Geometry check sheet. Reference: the model listing, model coordinates, mm. A direction names the side the tool comes from. Give positions to 0.01 mm unless a question says otherwise; leave off trailing zeros. Loops run counter-clockwise (first coordinate to the right, second up) from the corner with the lowest first, then second, coordinate; pieces in that order, holes last. Notation, with made-up numbers: (30, -0.5) -> (47, -0.5) arc R11 ccw to (47, 8.5) -> close; hole circle Ø9 at (53, 74.5). An arc over 180 degrees is marked (long way). One line per item, written item: value. Start each with the question number.
(1) Sectioned sample at B-B, the plane y = 25. Record the cut outline in (x, z).
(2) Sectioned sample at C-C, the plane z = 0. Record the cut outline in (x, y), then the cut area to 3 significant figures.
(3) Tool access check on faces 1 (the face through (0, 29, -16)), 2 (the face through (-22.7, 29.7, -10)), 3 (the face through (36, 8, 7.276)). Record the directions out of +Z, -Z, +X, -X, +Y, -Y that give a thin tool (end or side, any length) a straight path to the whole face; none if there is none.
(4) Scan lines: line 1 along Z through (x, y) = (-13, 40); line 2 along X through (y, z) = (40, -16.5); line 3 along Y through (x, z) = (-24, 14.5). Record each from-to range of solid material in increasing order. Write a range as from..to.
(5) Sectioned sample at A-A, the plane x = -24. Record the cut outline in (y, z).
(6) Gauge pin test, flat ends, axial feed: pin 1 Ø9.5 at (y, z) = (32.5, -14.5) entering from +X; pin 2 Ø2 at (x, z) = (-1, -11) entering from +Y; pin 3 Ø2 at (x, z) = (29.5, 10) entering from +Y; pin 4 Ø8 at (y, z) = (27, -3.5) entering from +X. Record the tip position at first contact, or that the pin passes through.
(7) Sectioned sample at D-D, the plane z = -19. Record the cut outline in (x, y).
(8) Draft check along X on faces 4 (the face through (-48, 15, 0)), 5 (the face through (12, 16, 0)), 6 (the face through (16.725, 7.888, 0.16)). Enter one of: pulls with the +X half, pulls with the -X half, needs draft (parallel to the pull), parting line crosses it, or undercut.
from build123d import *

# Parameters (mm, degrees)
BOSS_EXTRUDE1_DEPTH = 16
CUT_EXTRUDE2_DEPTH  = 16
SKETCH3_R           = 10
BOSS_EXTRUDE2_DEPTH = 12
BOSS_EXTRUDE3_START = -12
SKETCH11_R          = 10
BOSS_EXTRUDE3_DEPTH = 12
FILLET1_R           = 2
FILLET2_R           = 2


with BuildPart() as part:
    # Sketch1 → Boss-Extrude1 (new body)
    with BuildSketch(Plane(origin=(0, 0, 0), x_dir=(1, 0, 0), z_dir=(0, 1, 0))):
        with BuildLine():
            Line((-48, 22), (48, 22))
            ThreePointArc((48, 22), (70, 0), (48, -22))
            Line((48, -22), (-48, -22))
            Line((-48, -22), (-48, 22))
        make_face()
    extrude(amount=BOSS_EXTRUDE1_DEPTH)

    # Sketch2 → Cut-Extrude2 (cut)
    with BuildSketch(Plane(origin=(0, 0, 0), x_dir=(1, 0, 0), z_dir=(0, 1, 0))):
        with BuildLine():
            Line((48, -7.276334806), (24, -7.276334806))
            ThreePointArc((24, -7.276334806), (16.723665194, 0), (24, 7.276334806))
            Line((24, 7.276334806), (48, 7.276334806))
            ThreePointArc((48, 7.276334806), (55.276334806, 0), (48, -7.276334806))
        make_face()
    extrude(amount=CUT_EXTRUDE2_DEPTH, mode=Mode.SUBTRACT)

    # Sketch3 → Boss-Extrude2 (add)
    with BuildSketch(Plane.XY.offset(22)):
        with BuildLine():
            Line((-48, 40), (-48, 16))
            Line((-48, 16), (0, 16))
            Line((0, 16), (0, 40))
            ThreePointArc((0, 40), (-24, 64), (-48, 40))
        make_face()
        with Locations((-24, 40)):
            Circle(SKETCH3_R, mode=Mode.SUBTRACT)
    extrude(amount=-BOSS_EXTRUDE2_DEPTH)

    # Sketch11 → Boss-Extrude3 (add)
    with BuildSketch(Plane(origin=(0, 0, -22), x_dir=(-1, 0, 0), z_dir=(0, 0, -1)).offset(BOSS_EXTRUDE3_START)):
        with BuildLine():
            Line((0, 16), (48, 16))
            Line((48, 16), (48, 40))
            ThreePointArc((48, 40), (24, 64), (0, 40))
            Line((0, 40), (0, 16))
        make_face()
        with Locations(Location((24, 40, 0), (0, 0, 180))):
            Circle(SKETCH11_R, mode=Mode.SUBTRACT)
    extrude(amount=BOSS_EXTRUDE3_DEPTH)

    # Fillet1
    fillet1_edges = [part.edges().sort_by_distance(p)[0] for p in [
        (0, 16, 16),
    ]]
    fillet(fillet1_edges, radius=FILLET1_R)

    # Fillet2
    fillet2_edges = [part.edges().sort_by_distance(p)[0] for p in [
        (0, 16, -16),
    ]]
    fillet(fillet2_edges, radius=FILLET2_R)


solid = part.part
Calculated:
1. outline: (-48, -22) -> (0, -22) -> (0, -10) -> (-48, -10) -> close; (-48, 10) -> (0, 10) -> (0, 22) -> (-48, 22) -> close
2. outline: (-48, 0) -> (16.72, 0) -> (16.72, 16) -> (-48, 16) -> close; (55.28, 0) -> (70, 0) -> (70, 16) -> (55.28, 16) -> close
2. area: 1,270 mm2
3. face 1: +Z, -Z, +X, +Y
3. face 2: +X, -X, +Y
3. face 3: +Y, -Y
4. line 1: z = -22..-10, 10..22
4. line 2: x = -48..-34, -14..0
4. line 3: y = 0..30, 50..64
5. outline: (0, -22) -> (30, -22) -> (30, -10) -> (16, -10) -> (16, 10) -> (30, 10) -> (30, 22) -> (0, 22) -> close; (50, -22) -> (64, -22) -> (64, -10) -> (50, -10) -> close; (50, 10) -> (64, 10) -> (64, 22) -> (50, 22) -> close
6. pin 1: stops at x = 0
6. pin 2: stops at y = 49.59
6. pin 3: stops at y = 16
6. pin 4: passes through
7. outline: (-48, 0) -> (59.09, 0) -> (59.09, 16) -> (2, 16) arc R2 cw to (0, 18) -> (0, 40) arc R24 ccw to (-48, 40) -> close; hole circle Ø20 at (-24, 40)
8. face 4: pulls with the -X half
8. face 5: needs draft
8. face 6: undercut
